```python
from build123d import *

# Parameters (mm, degrees)
BASE_DEPTH               = 5
ESQUISSE8_R              = 5
ENL_V_MAT_EXTRU_7_DEPTH  = 10
ESQUISSE4_R              = 11
ESQUISSE4_R_2            = 3.5
ESQUISSE4_RX             = 1.5
ESQUISSE4_RY             = 0.5
ESQUISSE4_W              = 20
ESQUISSE4_H              = 14
ENL_V_MAT_EXTRU_8_DEPTH  = 10
ESQUISSE2_R              = 3
ESQUISSE2_R_2            = 2.5
ENL_V_MAT_EXTRU_9_DEPTH  = 10
ESQUISSE11_R             = 1.5
ENL_V_MAT_EXTRU_11_DEPTH = 5


with BuildPart() as part:
    # Esquisse1 → Base (new body)
    with BuildSketch(Plane.XY):
        Polygon((0, 0), (-175, 0), (-199.748737342, 24.748737342), (-199.748737342, 244.748737342), (-175, 269.497474683), (0, 269.497474683), (24.748737342, 244.748737342), (24.748737342, 24.748737342), align=None)
    extrude(amount=BASE_DEPTH)

    # Esquisse8 → Enlèv. mat.-Extru.7 (cut)
    with BuildSketch(Plane.XY.offset(5)):
        with Locations((-120.5, 256.997474683)):
            Circle(ESQUISSE8_R)
    extrude(amount=-ENL_V_MAT_EXTRU_7_DEPTH, mode=Mode.SUBTRACT)

    # Esquisse4 → Enlèv. mat.-Extru.8 (cut)
    with BuildSketch(Plane.XY.offset(5)):
        with Locations((-87.5, 234.497474683)):
            Circle(ESQUISSE4_R)
        with Locations((-137.5, 234.497474683)):
            Circle(ESQUISSE4_R_2)
        with Locations((-37.5, 234.497474683)):
            Circle(ESQUISSE4_R_2)
        with Locations(Location((-103.5, 256.997474683), (0, 0, -90))):
            Ellipse(ESQUISSE4_RX, ESQUISSE4_RY)
        with Locations(Location((-87.5, 256.997474683), (0, 0, -90))):
            Ellipse(ESQUISSE4_RX, ESQUISSE4_RY)
        with Locations(Location((-71.5, 256.997474683), (0, 0, -90))):
            Ellipse(ESQUISSE4_RX, ESQUISSE4_RY)
        with Locations(Location((-55.5, 256.997474683), (0, 0, -90))):
            Ellipse(ESQUISSE4_RX, ESQUISSE4_RY)
        with Locations((-87.5, 211.748737342)):
            Rectangle(ESQUISSE4_W, ESQUISSE4_H)
    extrude(amount=-ENL_V_MAT_EXTRU_8_DEPTH, mode=Mode.SUBTRACT)

    # Esquisse2 → Enlèv. mat.-Extru.9 (cut)
    with BuildSketch(Plane.XY.offset(5)):
        with Locations((-141.998737342, 12.5)):
            Circle(ESQUISSE2_R)
        with Locations((-141.998737342, 256.997474683)):
            Circle(ESQUISSE2_R)
        with Locations((-33.001262658, 12.5)):
            Circle(ESQUISSE2_R)
        with Locations((-33.001262658, 256.997474683)):
            Circle(ESQUISSE2_R)
        with Locations((-137.5, 123.748737342)):
            Circle(ESQUISSE2_R_2)
        with Locations((-126.5, 184.748737342)):
            Circle(ESQUISSE2_R_2)
        with Locations((-37.5, 123.748737342)):
            Circle(ESQUISSE2_R_2)
        with Locations((-48.5, 184.748737342)):
            Circle(ESQUISSE2_R_2)
    extrude(amount=-ENL_V_MAT_EXTRU_9_DEPTH, mode=Mode.SUBTRACT)

    # Esquisse11 → Enlèv. mat.-Extru.11 (cut)
    with BuildSketch(Plane.XY.offset(5)):
        with Locations((-170.614939475, 118.152371839)):
            Circle(ESQUISSE11_R)
        with Locations((-128.614939475, 61.152371839)):
            Circle(ESQUISSE11_R)
        Polygon((-189.748737342, -12.261016229), (-189.748737342, 134.748737342), (-189.748737342, 274.920827955), (-199.748737342, 274.920827955), (-199.748737342, -12.261016229), align=None)
    extrude(amount=-ENL_V_MAT_EXTRU_11_DEPTH, mode=Mode.SUBTRACT)


solid = part.part
```
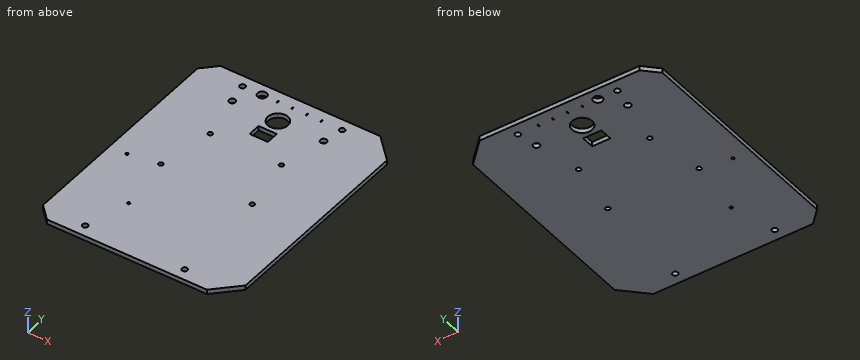
Check sheet for the modelled part. Datum: model origin and axes. Units: mm. Give positions to 0.01 mm unless a question says otherwise; leave off trailing zeros. Write each loop counter-clockwise with the first axis right and the second up, starting at its lowest first coordinate (ties: lowest second). Pieces come first, ordered by that corner, then holes.
Item 1: Cross-section at A-A (x = -120.5). Enter the section's corners in (y, z).
Item 2: Cross-section at B-B (z = 2.5). Count the separate pieces of the cut face and the enclosed holes in it, and give its area (3 significant figures).
Item 3: Scan lines: L1, parallel to Y at x = -37.5, z = 2.2; L2, parallel to X at y = 231.5, z = 4.15; L3, parallel to Y at x = -126.5, z = 1.05. Record each from-to range of solid material in increasing order.
Report:
1. outline: (0, 0) - (252, 0) - (252, 5) - (0, 5) - close; (262, 0) - (269.5, 0) - (269.5, 5) - (262, 5) - close
2. separate pieces: 1
2. enclosed holes: 19
2. area: 55,900 mm2
3. L1: y = 0 to 121.25, 126.25 to 231, 238 to 269.5
3. L2: x = -189.75 to -139.31, -135.69 to -98.08, -76.92 to -39.31, -35.69 to 24.75
3. L3: y = 0 to 182.25, 187.25 to 269.5
